Input: dimensioned drawing with shaded views. Units: mm. Origin: part minimum x, y, z. A direction names the side the tool comes from. Give positions to 0.01 mm unless a question says otherwise; leave off trailing zeros. Loops run counter-clockwise (first coordinate to the right, second up) from the corner with the lowest first, then second, coordinate; pieces in that order, holes last.
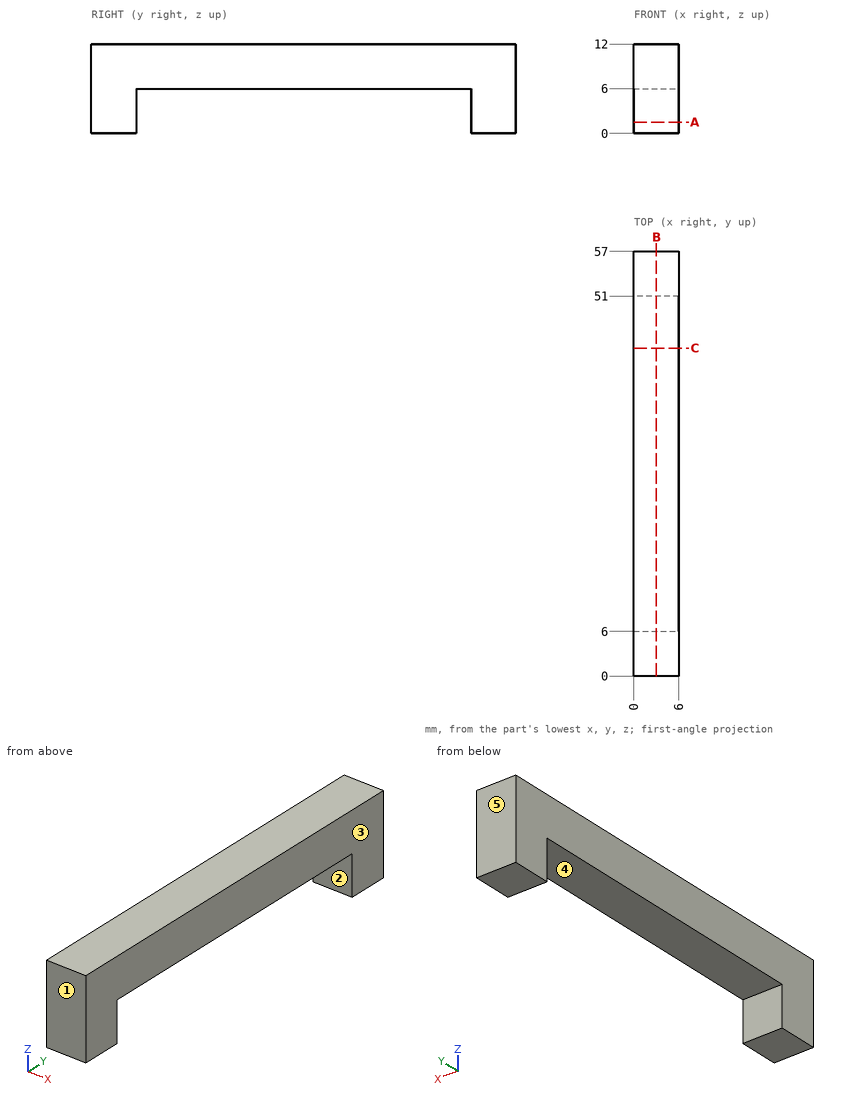
(1) First-contact query: pin 1 (1 mm diameter, centred on x = 3, z = 7, fed in from -Y); pin 2 (3 mm diameter, centred on x = 5, y = 23, fed in from -Z). Flat tips, straight axial feed; report the tip coordinate or a pass-through.
A:
pin 1: stops at y = 0
pin 2: stops at z = 6
(2) Reachability of the marked faces 1 and 2 from +Z, -Z, +X, -X, +Y, -Y: full face, straight path, thin tool, end or side. Return the list, or none.
A:
face 1: +Z, -Z, +X, -X, -Y
face 2: -Z, +X, -X
(3) Ray query, line 1 along Y through (x, z) = (0.75, 1.5); line 2 along Z through (x, y) = (3.5, 47). Return the intervals inside material, ascending.
A:
line 1: y = 0 to 6, 51 to 57
line 2: z = 6 to 12
(4) Mould query, pull axis Y, two halves, no side actions, for the marked faces 3, 4 and 5. Classes: pulls with the +Y half, pulls with the -Y half, needs draft (parallel to the pull), parting line crosses it, or undercut.
A:
face 3: needs draft
face 4: undercut
face 5: pulls with the +Y half
(5) Section A-A, the plane z = 1.5. Return the cut outline in (x, y), then the cut area to 3 significant figures.
A:
outline: (0, 0) - (6, 0) - (6, 6) - (0, 6) - close; (0, 51) - (6, 51) - (6, 57) - (0, 57) - close
area: 72.0 mm2
(6) Section B-B, the plane x = 3. Return the cut outline in (y, z), then the cut area to 3 significant figures.
A:
outline: (0, 0) - (6, 0) - (6, 6) - (51, 6) - (51, 0) - (57, 0) - (57, 12) - (0, 12) - close
area: 414 mm2
(7) Section C-C, the plane y = 44. Return the cut outline in (x, z).
A:
outline: (0, 6) - (6, 6) - (6, 12) - (0, 12) - close
